Autodesk Inventor part; units mm, degrees
ref_plane "YZ Plane" through (0, 0, 0) normal (1, 0, 0) x (0, 1, 0)
ref_plane "XZ Plane" through (0, 0, 0) normal (0, 1, 0) x (-1, 0, 0)
ref_plane "XY Plane" through (0, 0, 0) normal (0, 0, 1) x (1, 0, 0)
sketch "Sketch2" plane through (0, 0, 0) normal (1, 0, 0) x (0, 1, 0)
  line L0 (45.0919, 116.9004) -> (15.0919, 116.9004)
  line L1 (15.0919, 116.9004) -> (15.0919, -73.0996)
  line L2 (15.0919, -73.0996) -> (45.0919, -73.0996)
  line L3 (45.0919, -73.0996) -> (45.0919, 116.9004)
  point P0 (0, 0)
  dimension "d0" = 30
  dimension "d1" = 190
extrude "Extrusion1" add sketch "Sketch2" along normal blind 3
sketch "Sketch4" plane through (0, 0, 0) normal (-1, 0, 0) x (0, 0, 1)
  circle A0 centre (-67.0996, 38.6968) radius 2
  line L0 (-73.0996, 15.0919) -> (-73.0996, 45.0919)
  point P0 (0, 0)
  dimension "d7" = 4
  dimension "d8" = 6
extrude "Extrusion3" cut sketch "Sketch4" against normal blind 1
sketch "Sketch5" plane through (1, 38.6968, -67.0996) normal (-1, 0, 0) x (0, 0, 1)
  circle A0 centre (0, 0) radius 1
  point P0 (67.0996, -38.6968)
  dimension "d11" = 2
extrude "Extrusion4" cut sketch "Sketch5" against normal blind 2
sketch "Sketch6" plane through (0, 0, 0) normal (-1, 0, 0) x (0, 0, 1)
  circle A0 centre (-67.0996, 28.6968) radius 1
  circle A1 centre (-67.0996, 28.6968) radius 2
  circle A2 centre (-67.0996, 38.6968) radius 2
  point P0 (0, 0)
  dimension "d14" = 2
  dimension "d15" = 4
  dimension "d17" = 10
extrude "Extrusion5" cut sketch "Sketch6" against normal blind 1 contours A0 | A1
sketch "Sketch7" plane through (1, 28.6968, -67.0996) normal (-1, 0, 0) x (0, 0, 1)
  circle A0 centre (0, 0) radius 1
  point P0 (67.0996, -28.6968)
  dimension "d20" = 2
extrude "Extrusion6" cut sketch "Sketch7" against normal blind 2
sketch "Sketch8" plane through (0, 106.1298, -18.9436) normal (-1, 0, 0) x (0, 1, 0)
  circle A0 centre (-67.4331, 38.6843) radius 2
  line L0 (-73.0996, 15.0919) -> (-73.5243, 45.0873)
  circle A1 centre (-67.4331, 48.156) radius 2
  point P0 (0, 0)
  dimension "d23" = 4
  dimension "d24" = 6
  dimension "d45" = 9.4717
  dimension "d46" = 9.4717
extrude "Extrusion7" cut sketch "Sketch8" against normal blind 1 contours A0
sketch "Sketch9" plane through (1, 38.6968, -57.6279) normal (-1, 0, 0) x (0, 0, 1)
  circle A0 centre (0, 0) radius 1
  point P0 (67.0996, -38.6968)
  dimension "d28" = 2
extrude "Extrusion8" cut sketch "Sketch9" against normal blind 2
sketch "Sketch10" plane through (0, 30.0919, 21.9004) normal (-1, 0, 0) x (0, -1, 0)
  circle A0 centre (1.395, -79.4792) radius 1
  circle A1 centre (1.395, -79.4792) radius 2
  circle A2 centre (-8.6049, -79.5283) radius 2
  circle A3 centre (1.3951, -89) radius 2
  point P0 (0, 0)
  dimension "d33" = 2
  dimension "d32" = 4
  dimension "d34" = 10
  dimension "d47" = 9.5208
  dimension "d48" = 9.5208
extrude "Extrusion9" cut sketch "Sketch10" against normal blind 1 contours A0 | A1
sketch "Sketch12" plane through (1, 28.6969, -57.5789) normal (-1, 0, 0) x (0, 0, 1)
  circle A0 centre (0, 0) radius 1
  point P0 (57.5789, -28.6969)
  dimension "d42" = 2
extrude "Extrusion11" cut sketch "Sketch12" against normal blind 2
sketch "Sketch14" plane through (0, -38.3101, -86.469) normal (-1, 0, 0) x (0, -1, 0)
  circle A0 centre (-67.007, 38.6968) radius 2
  line L0 (-73.0996, 15.0919) -> (-72.982, 45.0906)
  circle A1 centre (-67.007, 28.8901) radius 2
  point P0 (0, 0)
  dimension "d49" = 4
  dimension "d50" = 6
  dimension "d71" = 9.8066
extrude "Extrusion12" cut sketch "Sketch14" against normal blind 1 contours A0
sketch "Sketch15" plane through (1, 28.6969, -47.7722) normal (-1, 0, 0) x (0, 0, 1)
  circle A0 centre (0, 0) radius 1
  point P0 (67.0996, -38.6968)
  dimension "d54" = 2
extrude "Extrusion13" cut sketch "Sketch15" against normal blind 2
sketch "Sketch16" plane through (0, 30.0919, 21.9004) normal (-1, 0, 0) x (0, -1, 0)
  circle A0 centre (-8.605, -69.6678) radius 1
  circle A1 centre (-8.605, -69.6678) radius 2
  circle A2 centre (1.395, -69.6726) radius 2
  circle A3 centre (-8.6049, -79.5283) radius 2
  circle A4 centre (1.395, -79.4792) radius 2
  point P0 (0, 0)
  dimension "d59" = 2
  dimension "d58" = 4
  dimension "d60" = 10
  dimension "d68" = 9.8605
  dimension "d69" = 9.8066
extrude "Extrusion14" cut sketch "Sketch16" against normal blind 1 contours A0 | A1
sketch "Sketch17" plane through (1, 38.6969, -47.7675) normal (-1, 0, 0) x (0, 0, 1)
  circle A0 centre (0, 0) radius 1
  point P0 (67.0996, -28.6968)
  dimension "d64" = 2
extrude "Extrusion15" cut sketch "Sketch17" against normal blind 2
fillet "Fillet1" radius 2 4 edges at (1.5, 45.0919, 116.9004) (1.5, 15.0919, 116.9004) (1.5, 45.0919, -73.0996) (1.5, 15.0919, -73.0996)
sketch "Sketch18" plane through (0, 0, 0) normal (-1, 0, 0) x (0, 0, 1)
  circle A0 centre (110.9004, 38.6968) radius 2
  line L0 (116.9004, 43.0919) -> (116.9004, 17.0919)
  point P0 (0, 0)
  dimension "d73" = 4
  dimension "d79" = 6
extrude "Extrusion16" cut sketch "Sketch18" against normal blind 1
sketch "Sketch19" plane through (1, 38.6968, 110.9004) normal (-1, 0, 0) x (0, 0, 1)
  circle A0 centre (0, 0) radius 1
  point P0 (-110.9004, -38.6968)
  dimension "d76" = 2
extrude "Extrusion17" cut sketch "Sketch19" against normal blind 2
sketch "Sketch21" plane through (0, 0, 0) normal (-1, 0, 0) x (0, 0, 1)
  circle A0 centre (110.9004, 28.6968) radius 1
  circle A1 centre (110.9004, 38.6968) radius 1
  point P0 (0, 0)
  dimension "d84" = 2
  dimension "d90" = 10
extrude "Extrusion19" cut sketch "Sketch21" against normal blind 3 contours A0
sketch "Sketch22" plane through (0, 0, 0) normal (-1, 0, 0) x (0, 0, 1)
  circle A0 centre (110.9004, 28.6968) radius 1
  circle A1 centre (110.9004, 28.6968) radius 2
  point P0 (0, 0)
  dimension "d87" = 4
extrude "Extrusion20" cut sketch "Sketch22" against normal blind 1
sketch "Sketch23" plane through (0, 0, 0) normal (-1, 0, 0) x (0, 0, 1)
  circle A0 centre (100.9004, 38.6968) radius 2
  circle A1 centre (110.9004, 38.6968) radius 1
  point P0 (0, 0)
  dimension "d93" = 10
extrude "Extrusion21" cut sketch "Sketch23" against normal blind 1 contours A0
sketch "Sketch24" plane through (0, 0, 0) normal (-1, 0, 0) x (0, 0, 1)
  circle A0 centre (100.9004, 28.6968) radius 2
  circle A1 centre (110.9004, 28.6968) radius 2
  point P0 (0, 0)
  dimension "d97" = 10
extrude "Extrusion22" cut sketch "Sketch24" against normal blind 1 contours A0
sketch "Sketch25" plane through (0, 0, 0) normal (-1, 0, 0) x (0, 0, 1)
  circle A0 centre (90.9004, 38.6968) radius 2
  circle A1 centre (100.9004, 38.6968) radius 2
  point P0 (0, 0)
  dimension "d98" = 10
sketch "Sketch26" plane through (1, 28.6968, 100.9004) normal (-1, 0, 0) x (0, 0, 1)
  point P0 (-100.9004, -28.6968)
sketch "Sketch27" plane through (0, 0, 0) normal (-1, 0, 0) x (0, 0, 1)
  circle A0 centre (90.9004, 28.6968) radius 2
  circle A1 centre (100.9004, 28.6968) radius 2
  point P0 (0, 0)
  dimension "d99" = 10
extrude "Extrusion23" cut sketch "Sketch25" against normal blind 1 contours A0
extrude "Extrusion24" cut sketch "Sketch27" against normal blind 1 contours A0
sketch "Sketch28" plane through (0, 0, 0) normal (-1, 0, 0) x (0, 0, 1)
  point P0 (0, 0)
sketch "Sketch29" plane through (1, 38.6968, 90.9004) normal (-1, 0, 0) x (0, 0, 1)
  circle A0 centre (0, 0) radius 1
  circle A1 centre (0, -10) radius 2
  circle A2 centre (0, -10) radius 1
  circle A3 centre (10, -10) radius 2
  circle A4 centre (10, -10) radius 1
  circle A5 centre (10, 0) radius 2
  circle A6 centre (10, 0) radius 1
  point P0 (-90.9004, -38.6968)
  dimension "d104" = 2
  dimension "d105" = 2
extrude "Extrusion25" cut sketch "Sketch29" against normal blind 2 contours A0 | A2 | A4 | A6
sketch "Sketch30" plane through (0, 0, 0) normal (-1, 0, 0) x (0, 0, 1)
  point P0 (0, 0)
sketch "Sketch31" plane through (0, 0, 0) normal (-1, 0, 0) x (0, 0, 1)
  line L0 (21.9004, 37.6669) -> (23.6324, 36.6669)
  line L1 (23.6324, 36.6669) -> (23.6324, 34.6669)
  line L2 (23.6324, 34.6669) -> (21.9004, 33.6669)
  line L3 (21.9004, 33.6669) -> (20.1683, 34.6669)
  line L4 (20.1683, 34.6669) -> (20.1683, 36.6669)
  line L5 (20.1683, 36.6669) -> (21.9004, 37.6669)
  line L6 (21.9004, 27.6669) -> (23.6324, 26.6669)
  line L7 (23.6324, 26.6669) -> (23.6324, 24.6669)
  line L8 (23.6324, 24.6669) -> (21.9004, 23.6669)
  line L9 (21.9004, 23.6669) -> (20.1683, 24.6669)
  line L10 (20.1683, 24.6669) -> (20.1683, 26.6669)
  line L11 (20.1683, 26.6669) -> (21.9004, 27.6669)
  point P0 (0, 0)
  point P1 (21.9004, 35.6669)
  point P2 (21.9004, 25.6669)
  dimension "d108" = 4
  dimension "d109" = 4
  dimension "d110" = 6
extrude "Extrusion26" cut sketch "Sketch31" against normal blind 1
sketch "Sketch32" plane through (1, 0, 0) normal (-1, 0, 0) x (0, 0, 1)
  circle A0 centre (21.9004, 25.6669) radius 1
  circle A1 centre (21.9004, 35.6669) radius 1
  point P0 (0, 0)
extrude "Extrusion27" cut sketch "Sketch32" against normal blind 2
sketch "Sketch33" plane through (0, 0, 0) normal (-1, 0, 0) x (0, 0, 1)
  circle A0 centre (-67.0996, 38.6968) radius 1
  line L0 (116.9004, 43.0919) -> (116.9004, 17.0919)
  point P0 (0, 0)
properties part number "Holder e Holder gripper"
Could you check a few things on this model? Use its own coordinates, in mm. Give positions to 0.01 mm unless a question says otherwise; leave off trailing zeros. One line per item, written item: value. Start each with the question number.
Item 1: If we mould it in two halves opening along Z, with no side actions, what happens to faces 1 (the face through (0.49, 40.05, 89.43)), 2 (the face through (1, 30, 116.9)), 3 (the face through (1, 30, -73.1))? For each: +Z half, -Z half, draft (parallel to the pull), parting line (faces both ways), or undercut.
Item 2: I'm going to push flat-ended pins straight in: pin 1 (1.6 mm diameter, centred on y = 25.67, z = 21.9, fed in from +X); pin 2 (2 mm diameter, centred on y = 38, z = -48, fed in from -X). Where does each tip first touch, or does it pass through?
Item 3: Please list where these lines run through material, in increasing order: line 1 (Y direction, x = 2.4, z = -58) (3 decimals); line 2 (Z direction, x = 2, y = 25). Write a range as from..to.
Geometry says:
1. face 1: undercut
1. face 2: +Z half
1. face 3: -Z half
2. pin 1: through
2. pin 2: x = 1
3. line 1: 15.092..27.79, 29.604..37.769, 39.625..45.092
3. line 2: -73.1..21.16, 22.65..116.9
